The model under review builds one solid part; all positions refer to its coordinate system, in mm. Face numbers are marked on the shaded views. A direction names the side the tool comes from. Coordinates: 2 decimals unless noted, no trailing zeros. Order: outer loops, then holes, each group sorted by start corner. A loop starts at its lowest first (then second) coordinate and runs counter-clockwise, first axis right, second up. Notation, with made-up numbers: M -19,88 L -10,88 A24 cw -10,127 Z; hole C 82.25,61.5 d9. An arc over 180 degrees is marked long. One line per item, written item: value.
```python
from build123d import *

# Parameters (mm, degrees)
F0_W     = 609.6
F0_H     = 609.6
F1_DEPTH = 914.4
F2_W     = 609.6
F2_H     = 609.6
F2_H_2   = 25.4
F3_DEPTH = 38.1
F4_W     = 609.6
F4_H     = 152.4
F4_W_2   = 208.593592
F4_H_2   = 29.799104
F5_DEPTH = 12.7
F6_W     = 406.4
F6_H     = 406.4
F7_DEPTH = 762


with BuildPart() as f1:
    # F0 (on Top) → F1 (new body)
    with BuildSketch(Plane.XY):
        Rectangle(F0_W, F0_H)
    extrude(amount=F1_DEPTH)

    # F2 (on face) → F3 (join)
    with BuildSketch(Plane.XY.offset(914.4)):
        Rectangle(F2_W, F2_H)
        with Locations((0, -317.5)):
            Rectangle(F2_W, F2_H_2)
    extrude(amount=-F3_DEPTH)

    # F4 (on face) → F5 (join)
    with BuildSketch(Plane.XZ.offset(304.8)):
        with Locations((0, 800.1)):
            Rectangle(F4_W, F4_H)
        with Locations((0, 809.027108)):
            Rectangle(F4_W_2, F4_H_2, mode=Mode.SUBTRACT)
    extrude(amount=F5_DEPTH)

    # F6 (on face) → F7 (cut)
    with BuildSketch(Plane(origin=(0, 0, 0), x_dir=(1, 0, 0), z_dir=(0, 0, -1))):
        Rectangle(F6_W, F6_H)
    extrude(amount=-F7_DEPTH, mode=Mode.SUBTRACT)


solid = f1.part
```
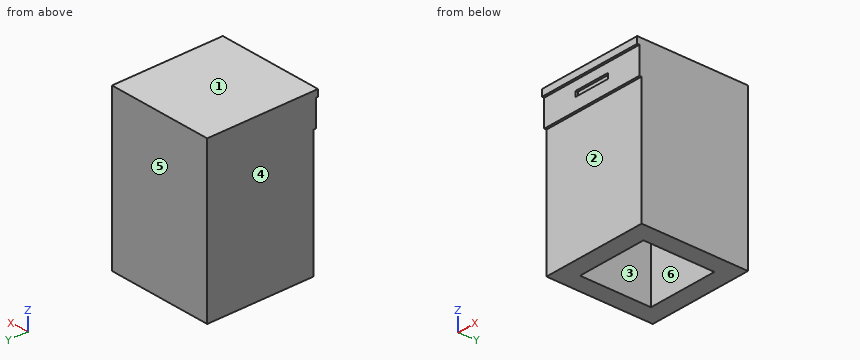
(1) We need section B-B, the plane y = 187. State the section outline as (x, z) points.
Geometry results:
outline: M -304.8,0 L -203.2,0 L -203.2,762 L 203.2,762 L 203.2,0 L 304.8,0 L 304.8,914.4 L -304.8,914.4 Z
(2) We need section A-A, the plane z = 519. State the section outline as (x, y) points.
Geometry results:
outline: M -304.8,-304.8 L 304.8,-304.8 L 304.8,304.8 L -304.8,304.8 Z; hole M -203.2,-203.2 L 203.2,-203.2 L 203.2,203.2 L -203.2,203.2 Z
(3) We need section D-D, the plane x = 8. State the section outline as (y, z) points.
Geometry results:
outline: M -330.2,876.3 L -317.5,876.3 L -317.5,823.93 L -304.8,823.93 L -304.8,794.13 L -317.5,794.13 L -317.5,723.9 L -304.8,723.9 L -304.8,0 L -203.2,0 L -203.2,762 L 203.2,762 L 203.2,0 L 304.8,0 L 304.8,914.4 L -330.2,914.4 Z
(4) Mouldability with a two-part tool opening along X and no side actions: class the marked faces 4, 5 and 6 as +X half, -X half, draft (parallel to the pull), parting line (faces both ways), or undercut.
Geometry results:
face 4: -X half
face 5: draft
face 6: undercut
(5) Tool access review of the marked faces 1, 2 and 3: name each direction out of +Z, -Z, +X, -X, +Y, -Y from which nothing blocks a thin tool from reaching the whole face with its end or side.
Geometry results:
face 1: +Z, +X, -X, +Y, -Y
face 2: -Z, +X, -X, -Y
face 3: -Z
(6) We need section C-C, the plane x = 159.5. State the section outline as (y, z) points, plus the area to 3 significant figures.
Geometry results:
outline: M -330.2,876.3 L -317.5,876.3 L -317.5,723.9 L -304.8,723.9 L -304.8,0 L -203.2,0 L -203.2,762 L 203.2,762 L 203.2,0 L 304.8,0 L 304.8,914.4 L -330.2,914.4 Z
area: 251,000 mm2
(7) Insertion check: pin 1 Ø15 at (x, z) = (-27.5, 808) entering from -Y; pin 2 Ø4 at (x, y) = (-56.5, -326) entering from -Z; pin 3 Ø12 at (x, y) = (-102, -170) entering from -Z. Each pin has a flat end and moves straight along its axis. Give the tip position at first contact, or say it passes through.
Geometry results:
pin 1: stops at y = -304.8
pin 2: stops at z = 876.3
pin 3: stops at z = 762
(8) For L1, parallel to X at y = -139, z = 374; L2, parallel to Z at x = -32, y = 4.5, list the stretches that pass through material, from the lowest coordinate up.
Geometry results:
L1: x = -304.8 to -203.2, 203.2 to 304.8
L2: z = 762 to 914.4
